Geometry: see drawing. Coordinates: mm, zero at the bounding-box minimum. A direction names the side the tool comes from. Round coordinates to 2 decimals unless told otherwise and drop trailing zeros. Loops run counter-clockwise (first coordinate to the right, second up) from the corner with the lowest first, then second, coordinate; pieces in that order, holes last. Notation, with made-up numbers: (82.25, 34) - (108.25, 34) arc R31 cw to (108.25, 58) - close; hole circle Ø1 at (36, 6). An arc over 180 degrees is marked (long way). Answer in a Markdown table with one row per item. Add a question column.
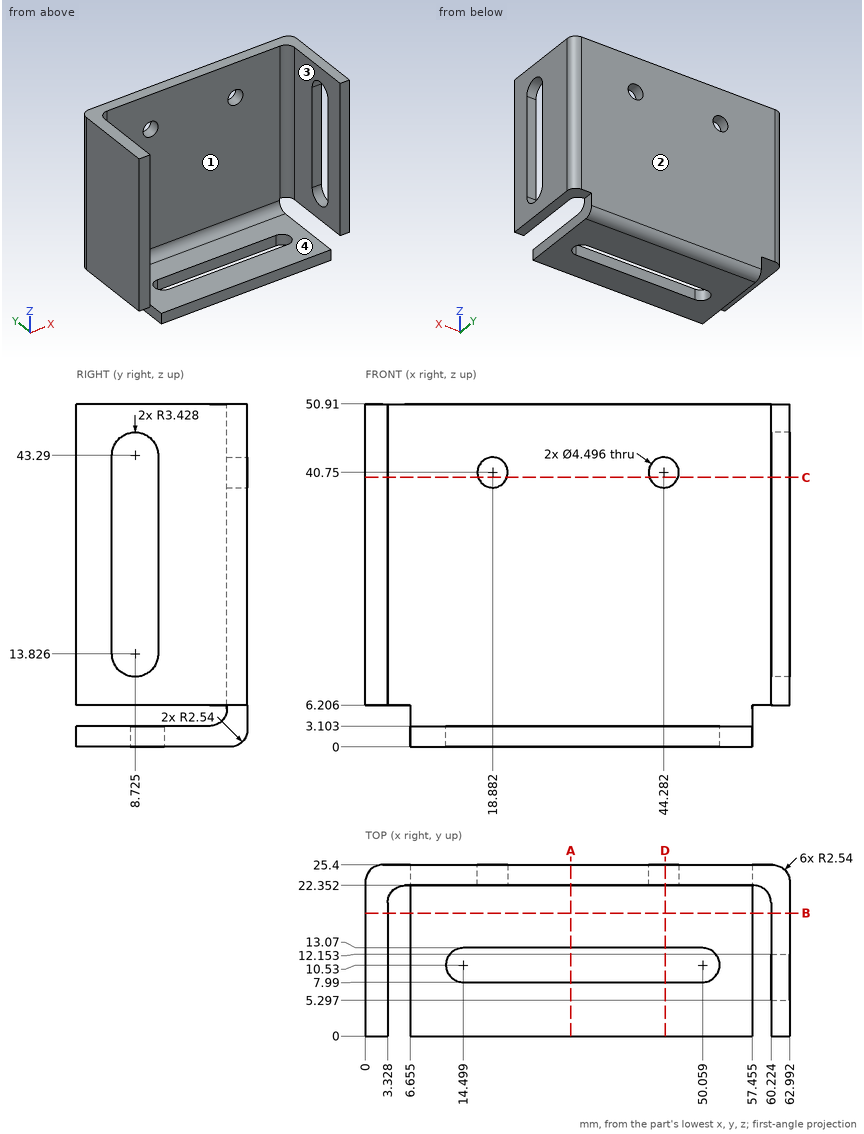
1) Reachability of the marked faces 1, 2, 3 and 4 from +Z, -Z, +X, -X, +Y, -Y: full face, straight path, thin tool, end or side. Return the list, or none.
2) Section B-B, the plane y = 18.25. Return the cut outline in (x, z) (1 decimal), and give its area (3 significant figures).
3) Section C-C, the plane z = 40. Return the cut outline in (x, y).
4) Material intervals for line 1 along X through (y, z) = (2.5, 16); line 2 along Z through (x, y) = (32, 7); line 3 along Y through (x, z) = (34.5, 36.5), sorted ascending. Write a range as from..to.
5) Section A-A, the plane x = 30.5. Return the cut outline in (y, z).
6) Contact query for flat-ended pins moving along their axis: pin 1 Ø3.5 at (x, y) = (1.5, 16.5) entering from -Z; pin 2 Ø1.9 at (y, z) = (13.5, 4) entering from -X (1 decimal); pin 3 Ø1 at (x, z) = (10, 9.5) entering from -Y; pin 4 Ø1.9 at (y, z) = (9, 4.5) entering from +X. Output: stop coordinate, or through.
7) Section D-D, the plane x = 44.5. Return the cut outline in (y, z).
Evaluation:
| question | item | result |
|---|---|---|
| 1 | face 1 | +Z, -Y |
| 1 | face 2 | +Z, -Z, +X, -X, +Y |
| 1 | face 3 | +Z, -Z, -Y |
| 1 | face 4 | +Z, +X, -X, -Y |
| 2 | outline | (0, 6.2) - (3.3, 6.2) - (3.3, 50.9) - (0, 50.9) - close; (6.7, 0) - (57.5, 0) - (57.5, 3.1) - (6.7, 3.1) - close; (60.2, 6.2) - (63, 6.2) - (63, 50.9) - (60.2, 50.9) - close |
| 2 | area | 430 mm² |
| 3 | outline | (0, 0) - (3.33, 0) - (3.33, 19.81) arc R2.54 cw to (5.87, 22.35) - (16.76, 22.35) - (16.76, 25.4) - (2.54, 25.4) arc R2.54 ccw to (0, 22.86) - close; (21, 22.35) - (42.16, 22.35) - (42.16, 25.4) - (21, 25.4) - close; (46.4, 22.35) - (57.68, 22.35) arc R2.54 cw to (60.22, 19.81) - (60.22, 12.15) - (62.99, 12.15) - (62.99, 22.86) arc R2.54 ccw to (60.45, 25.4) - (46.4, 25.4) - close; (60.22, 0) - (62.99, 0) - (62.99, 5.3) - (60.22, 5.3) - close |
| 4 | line 1 | x = 0..3.33, 60.22..62.99 |
| 4 | line 2 | z = 0..3.1 |
| 4 | line 3 | y = 22.35..25.4 |
| 5 | outline | (0, 0) - (7.99, 0) - (7.99, 3.1) - (0, 3.1) - close; (13.07, 0) - (22.86, 0) arc R2.54 ccw to (25.4, 2.54) - (25.4, 50.91) - (22.35, 50.91) - (22.35, 5.64) arc R2.54 cw to (19.81, 3.1) - (13.07, 3.1) - close |
| 6 | pin 1 | stops at z = 6.21 |
| 6 | pin 2 | stops at x = 6.7 |
| 6 | pin 3 | stops at y = 22.35 |
| 6 | pin 4 | passes through |
| 7 | outline | (0, 0) - (7.99, 0) - (7.99, 3.1) - (0, 3.1) - close; (13.07, 0) - (22.86, 0) arc R2.54 ccw to (25.4, 2.54) - (25.4, 38.51) - (22.35, 38.51) - (22.35, 5.64) arc R2.54 cw to (19.81, 3.1) - (13.07, 3.1) - close; (22.35, 42.99) - (25.4, 42.99) - (25.4, 50.91) - (22.35, 50.91) - close |
